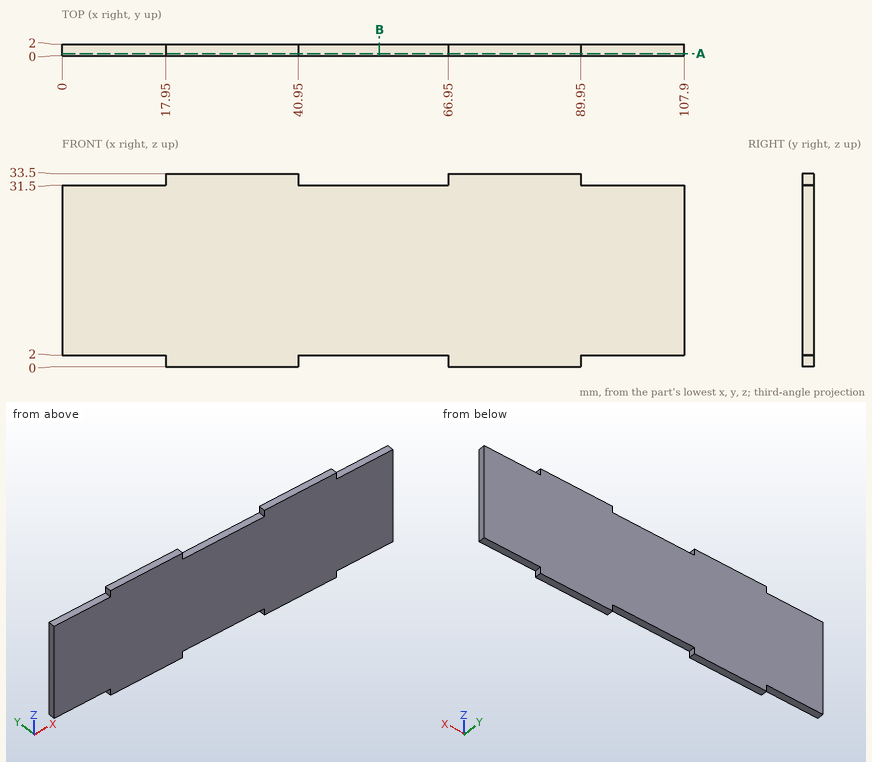
Print and shaded views of the part. All mm, measured from the part's lowest x, y and z. Give positions to 0.01 mm unless a question says otherwise; leave off trailing zeros. Write each loop counter-clockwise with the first axis right and the second up, starting at its lowest first coordinate (ties: lowest second). Pieces come first, ordered by that corner, then holes. Notation, with made-up numbers: (20.25, 77.5) - (51.25, 77.5) arc R31 cw to (51.25, 104.5) - close; hole circle Ø3 at (-4.5, 13). An arc over 180 degrees is marked (long way). Put each result on its own line as item: value.
(1) Saw through at A-A (y = 0.35). List the corners of the cut face in (x, z).
Working result:
outline: (0, 2) - (17.95, 2) - (17.95, 0) - (40.95, 0) - (40.95, 2) - (66.95, 2) - (66.95, 0) - (89.95, 0) - (89.95, 2) - (107.9, 2) - (107.9, 31.5) - (89.95, 31.5) - (89.95, 33.5) - (66.95, 33.5) - (66.95, 31.5) - (40.95, 31.5) - (40.95, 33.5) - (17.95, 33.5) - (17.95, 31.5) - (0, 31.5) - close
(2) Saw through at B-B (x = 55). List the corners of the cut face in (y, z), then the cut area to 3 significant figures.
Working result:
outline: (0, 2) - (2, 2) - (2, 31.5) - (0, 31.5) - close
area: 59.0 mm^2
(3) Wall check: L1, parallel to Z at x = 7.5, y = 0.45. Give the ranges that are in metal, low to high.
Working result:
L1: 2 to 31.5
(4) Drop flat-ended pins along their axis: pin 1 Ø0.6 at (x, y) = (11, 1) entering from -Z; pin 2 Ø5 at (x, z) = (31.5, 6.5) entering from -Y; pin 3 Ø0.6 at (x, y) = (102.5, 0.5) entering from +Z; pin 4 Ø1 at (y, z) = (1, 1) entering from +X. Give the stop position or say it passes through.
Working result:
pin 1: z = 2
pin 2: y = 0
pin 3: z = 31.5
pin 4: x = 89.95
